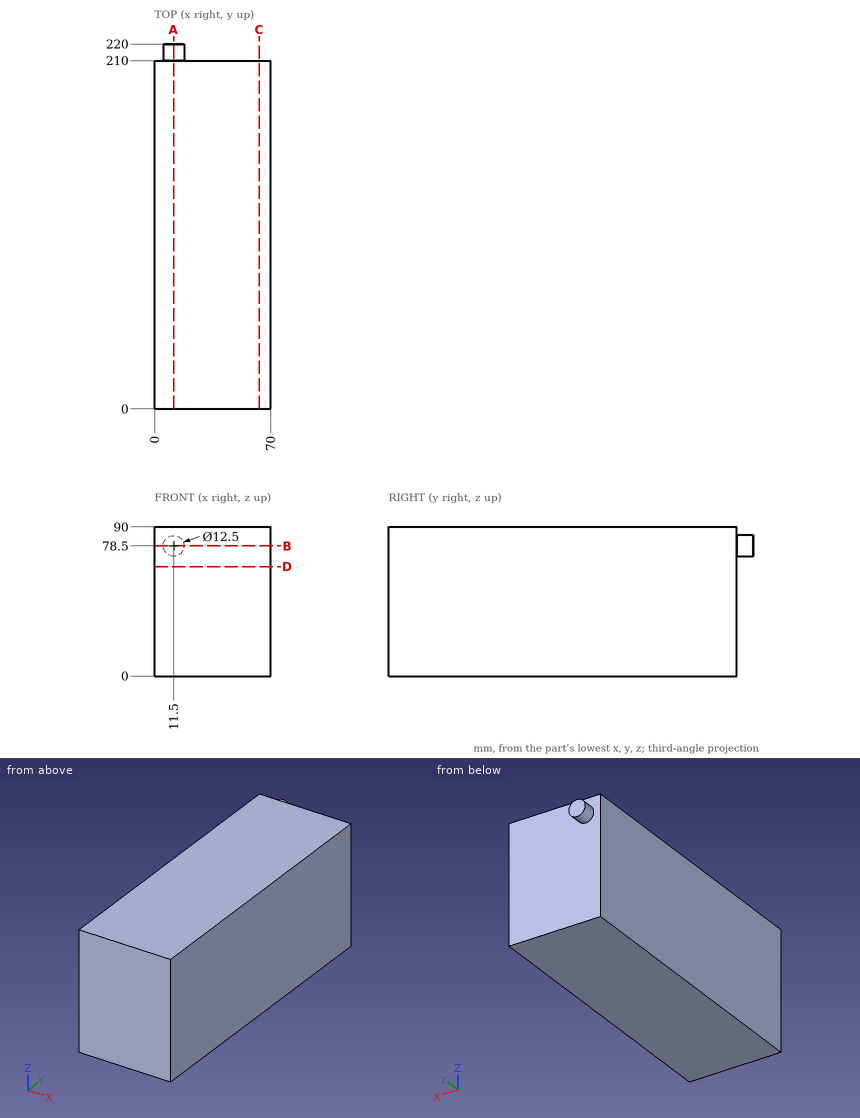
For this review, use the dimensioned drawing (mm, ordinates from the lowest corner) and the shaded views. Round coordinates to 2 decimals unless told otherwise and drop trailing zeros. Write each loop counter-clockwise with the first axis right and the second up, starting at its lowest first coordinate (ties: lowest second). Pieces come first, ordered by that corner, then holes. Notation, with made-up numbers: (79.5, 40) - (88.5, 40) arc R21 ccw to (88.5, 45) - close; hole circle Ø7 at (76.5, 73). An arc over 180 degrees is marked (long way). Use a Markdown table: item, result.
Q1. We need section C-C (x = 63). Give the boundary of the cut face in (y, z), plus the area to 3 significant figures.
Derived:
| item | result |
|---|---|
| outline | (0, 0) - (210, 0) - (210, 90) - (0, 90) - close |
| area | 18,900 mm2 |
Q2. Wall thickness on line 1 along Y through (x, z) = (13, 26): over which ranges is the line inside the solid? List them lowest first.
Derived:
| item | result |
|---|---|
| line 1 | y = 0 to 210 |
Q3. We need section D-D (z = 66). Give the boundary of the cut face in (x, y), plus the area to 3 significant figures.
Derived:
| item | result |
|---|---|
| outline | (0, 0) - (70, 0) - (70, 210) - (0, 210) - close |
| area | 14,700 mm2 |
Q4. We need section A-A (x = 11.5). Give the boundary of the cut face in (y, z), plus the area to 3 significant figures.
Derived:
| item | result |
|---|---|
| outline | (0, 0) - (210, 0) - (210, 72.25) - (220, 72.25) - (220, 84.75) - (210, 84.75) - (210, 90) - (0, 90) - close |
| area | 19,000 mm2 |
Q5. Clearance check with a flat-ended pin moving along its axis: pin 1 (1 mm diameter, centred on x = 31, z = 38, fed in from +Y). State where the tip first meets the part, or that it passes through.
Derived:
| item | result |
|---|---|
| pin 1 | stops at y = 210 |
Q6. We need section B-B (z = 78.5). Give the boundary of the cut face in (x, y).
Derived:
| item | result |
|---|---|
| outline | (0, 0) - (70, 0) - (70, 210) - (17.75, 210) - (17.75, 220) - (5.25, 220) - (5.25, 210) - (0, 210) - close |
